Geometry check sheet. Reference: the model listing, model coordinates, mm. Face numbers are marked on the shaded views. A direction names the side the tool comes from. Give positions to 0.01 mm unless a question says otherwise; leave off trailing zeros. Order: outer loops, then holes, each group sorted by start corner. A loop starts at its lowest first (then second) coordinate and runs counter-clockwise, first axis right, second up. Notation, with made-up numbers: M 23,13.5 L 69,13.5 A25 cw 69,25.5 Z; hole C -24.75,40 d11. An arc over 180 degrees is marked long. Answer as a JSON object with one key per item and string values. Group by question number.
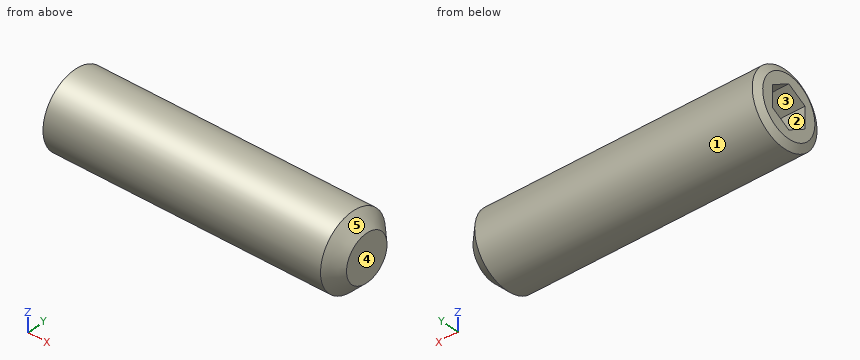
from build123d import *

# Parameters (mm, degrees)
HEX_2_DEPTH = 2.5


with BuildPart() as part:
    # BodySke → BaseBody (revolve)
    with BuildSketch(Plane.XY, mode=Mode.PRIVATE) as basebody_sk:
        Polygon((0, 0), (0, 1.61), (0.225166605, 2), (15.25, 2), (16, 1.25), (16, 0), align=None)
    revolve(basebody_sk.sketch.rotate(Axis((-12.7, 0, 0), (1, 0, 0)), 90), axis=Axis((-12.7, 0, 0), (1, 0, 0)))  # turned: the seam where the file's is

    # Sketch2 → Hex 2 (cut)
    with BuildSketch(Plane.ZY):
        Polygon((0.577350269, 1), (-0.577350269, 1), (-1.154700538, 0), (-0.577350269, -1), (0.577350269, -1), (1.154700538, 0), align=None)
    extrude(amount=-HEX_2_DEPTH, mode=Mode.SUBTRACT)


solid = part.part
1. Cross-section at A-A (z = 0). Record the cut outline in (x, y).
2. Cross-section at B-B (x = 13.75). Record the cut outline in (y, z), and give its area (3 significant figures).
3. Release check for a two-part mould opening along Y. For the marked faces 3, 4 and 5 record: released by +Y, released by -Y, zero draft, split by the parting line, or undercut.
4. Depth check by flat-ended pin: pin 1 (1.5 mm diameter, centred on x = 6.5, z = 0.5, fed in from +Y). Enter the tip coordinate at first touch or a pass-through.
5. Thickness scan on line 1 along X through (y, z) = (-0.7, 0.15); line 2 along Z through (x, y) = (1.25, 0.65); line 3 along X through (y, z) = (-1.35, 0.7). Record the ranges inside material, lowest first. Write a range as [from, to].
6. Access from +Z, -Z, +X, -X, +Y, -Y to the whole of each face (thin tool, end or side, straight path). Record for the marked faces 1 and 2.
Report:
{
 "1": {"outline": "M 0,-1.61 L 0.23,-2 L 15.25,-2 L 16,-1.25 L 16,1.25 L 15.25,2 L 0.23,2 L 0,1.61 L 0,1 L 2.5,1 L 2.5,-1 L 0,-1 Z"},
 "2": {"outline": "C 0,0 d4", "area": "12.6 mm2"},
 "3": {"face 3": "undercut", "face 4": "zero draft", "face 5": "split by the parting line"},
 "4": {"pin 1": "stops at y = 2"},
 "5": {"line 1": "x = [2.5, 16]", "line 2": "z = [-1.89, -0.78], [0.78, 1.89]", "line 3": "x = [0, 15.73]"},
 "6": {"face 1": "+X, -X", "face 2": "-X"}
}
